```python
from build123d import *

# Parameters (mm, degrees)
SKETCH_1_W                  = 80
SKETCH_1_H                  = 465
EXTRUDE_1_DEPTH             = 107
CUT_EXTRUDE_1_REACH         = 270.152
SKETCH_2_W                  = 45.5
SKETCH_2_H                  = 90
CUT_EXTRUDE_2_REACH         = 270.152
CUT_EXTRUDE_3_REACH         = 261.047
SKETCH_4_R                  = 20
HOLE_WIZARD_M8_1_D          = 6.8
HOLE_WIZARD_M8_1_DEPTH      = 17.25
CUT_EXTRUDE_4_REACH         = 261.047
SKETCH_8_R                  = 9
PATTERN_LINEAR_1_COUNT      = 2
PATTERN_LINEAR_1_PITCH      = 40
PATTERN_LINEAR_1_COUNT_DIR2 = 3
PATTERN_LINEAR_1_PITCH_DIR2 = 110
SKETCH_9_W                  = 80
SKETCH_9_H                  = 20
CUT_EXTRUDE_5_DEPTH         = 6.5
HOLE_WIZARD_M8_2_D          = 6.8
HOLE_WIZARD_M8_2_DEPTH      = 25
HOLE_WIZARD_M8_2_TIP        = 2.042926105
FILLET_1_R                  = 8


with BuildPart() as part:
    # 草图1 → 凸台-拉伸1 (new body)
    with BuildSketch(Plane.XY):
        Rectangle(SKETCH_1_W, SKETCH_1_H)
    extrude(amount=EXTRUDE_1_DEPTH)

    # 草图2 → 切除-拉伸1 (cut, up to next)
    with BuildSketch(Plane.ZY.offset(40), mode=Mode.PRIVATE) as cut_extrude_1_sk1:
        with BuildLine():
            Line((27, 232.5), (27, 115.5))
            ThreePointArc((27, 115.5), (24.656854249, 109.843145751), (19, 107.5))
            Line((19, 107.5), (0, 107.5))
            Line((0, 107.5), (0, 232.5))
            Line((0, 232.5), (27, 232.5))
        make_face()
    cut_extrude_1_tool1 = extrude(cut_extrude_1_sk1.sketch, amount=-CUT_EXTRUDE_1_REACH, mode=Mode.PRIVATE) & part.part
    # 草图2 → 切除-拉伸1 (cut, up to next)
    with BuildSketch(Plane.ZY.offset(40), mode=Mode.PRIVATE) as cut_extrude_1_sk2:
        with Locations((67, 187.5)):
            Rectangle(SKETCH_2_W, SKETCH_2_H)
    cut_extrude_1_tool2 = extrude(cut_extrude_1_sk2.sketch, amount=-CUT_EXTRUDE_1_REACH, mode=Mode.PRIVATE) & part.part
    add(cut_extrude_1_tool1.solids().sort_by_distance((-40, 170.248081, 13.452139))[0], mode=Mode.SUBTRACT)
    add(cut_extrude_1_tool2.solids().sort_by_distance((-40, 187.5, 67))[0], mode=Mode.SUBTRACT)

    # 草图3 → 切除-拉伸2 (cut, up to next)
    with BuildSketch(Plane.ZY.offset(40), mode=Mode.PRIVATE) as cut_extrude_2_sk1:
        Polygon((107, 119.530661885), (61.277191914, 42.311924553), (61.277191914, -232.5), (107, -232.5), align=None)
    cut_extrude_2_tool1 = extrude(cut_extrude_2_sk1.sketch, amount=-CUT_EXTRUDE_2_REACH, mode=Mode.PRIVATE) & part.part
    add(cut_extrude_2_tool1.solids().sort_by_distance((-40, -74.996659, 85.077337))[0], mode=Mode.SUBTRACT)

    # 切除-拉伸3: up to this face of the body (flat: up to its plane)
    cut_extrude_3_end = Plane(part.part.faces().sort_by_distance((0, 174, 27))[0])
    # 草图4 → 切除-拉伸3 (cut, up to the picked face)
    with BuildSketch(Plane.XY.offset(107), mode=Mode.PRIVATE) as cut_extrude_3_sk1:
        with Locations(Location((0, 192.5, 0), (0, 0, 270))):
            Circle(SKETCH_4_R)
    cut_extrude_3_tool1 = split(extrude(cut_extrude_3_sk1.sketch, amount=-CUT_EXTRUDE_3_REACH, mode=Mode.PRIVATE), bisect_by=cut_extrude_3_end, keep=Keep.BOTH, mode=Mode.PRIVATE)
    add(cut_extrude_3_tool1.solids().sort_by(Axis((0, 192.5, 107), (0, 0, -1)))[0], mode=Mode.SUBTRACT)

    # M8 螺纹孔1
    with Locations(Plane.XY.offset(107)):
        with Locations((-25, 162.5), (25, 162.5)):
            Hole(HOLE_WIZARD_M8_1_D / 2, depth=HOLE_WIZARD_M8_1_DEPTH)

    # 草图8 → 切除-拉伸4 (cut, up to next)
    with BuildSketch(Plane(origin=(0, 0, 0), x_dir=(-1, 0, 0), z_dir=(0, 0, -1)), mode=Mode.PRIVATE) as cut_extrude_4_sk1:
        with Locations((-20, 47.5)):
            Circle(SKETCH_8_R)
    cut_extrude_4_tool1 = extrude(cut_extrude_4_sk1.sketch, amount=-CUT_EXTRUDE_4_REACH, mode=Mode.PRIVATE) & part.part
    cut_extrude_4 = cut_extrude_4_tool1.solids().sort_by_distance((20, 47.5, 0))[0]
    add(cut_extrude_4, mode=Mode.SUBTRACT)

    # 阵列(线性)1: Cut-Extrude 4 2 × 3
    with Locations(*[(-i * PATTERN_LINEAR_1_PITCH, -j * PATTERN_LINEAR_1_PITCH_DIR2, 0) for i in range(PATTERN_LINEAR_1_COUNT) for j in range(PATTERN_LINEAR_1_COUNT_DIR2) if (i, j) != (0, 0)]):
        add(cut_extrude_4, mode=Mode.SUBTRACT)

    # 草图9 → 切除-拉伸5 (cut)
    with BuildSketch(Plane(origin=(0, 0, 0), x_dir=(-1, 0, 0), z_dir=(0, 0, -1))):
        with Locations((0, -117.5)):
            Rectangle(SKETCH_9_W, SKETCH_9_H)
    extrude(amount=-CUT_EXTRUDE_5_DEPTH, mode=Mode.SUBTRACT)

    # M8 螺纹孔2
    with Locations(Plane(origin=(0, 0, 6.5), x_dir=(-1, 0, 0), z_dir=(0, 0, -1))):
        with Locations((-20, -117.5), (20, -117.5)):
            Hole(HOLE_WIZARD_M8_2_D / 2, depth=HOLE_WIZARD_M8_2_DEPTH)
            with Locations((0, 0, -(HOLE_WIZARD_M8_2_DEPTH + HOLE_WIZARD_M8_2_TIP / 2))):  # 118° drill point
                Cone(0, HOLE_WIZARD_M8_2_D / 2, HOLE_WIZARD_M8_2_TIP, mode=Mode.SUBTRACT)

    # 圆角1
    fillet_1_edges = [part.edges().sort_by_distance(p)[0] for p in [
        (0, 142.5, 89.75),
        (0, 142.5, 44.25),
    ]]
    fillet(fillet_1_edges, radius=FILLET_1_R)


solid = part.part
```
Design review of the part built by this model. Coordinates are the model's own, in mm. A direction names the side the tool comes from. Give positions to 0.01 mm unless a question says otherwise; leave off trailing zeros. Write each loop counter-clockwise with the first axis right and the second up, starting at its lowest first coordinate (ties: lowest second). Pieces come first, ordered by that corner, then holes. Notation, with made-up numbers: (28, 83.5) - (35, 83.5) arc R30 ccw to (35, 119.5) - close; hole circle Ø1 at (-14, 6). An arc over 180 degrees is marked (long way). Return JSON: item names as keys, results as strings. Group by question number.
(1) Machinability: for faces 1 (the flat face through (-1, 107.5, 10)), 2 (the cylindrical face through (0.56, 144.781, 87.344)), 3 (the cylindrical face through (0.88, 212.48, 35.75)), 4 (the flat face through (-1, -93, 61.277)), 5 (the flat face through (40, -3, 41)), which of the approach directions +Z, -Z, +X, -X, +Y, -Y give a long, thin tool a straight path to every point of the face, cutting with its end or side? Answer none if there is none.
(2) We need section B-B, the plane z = 56.5. Give the boundary of the cut face in (x, y).
(3) To check wall thickness, follow probe 1 along X at (y, z) = (162, 95); probe 2 along Y at (x, z) = (-19.5, 11.5); probe 3 along X at (y, z) = (47.5, 45.5). State the ranges of each line that lie inside material, in increasing order.
(4) We need section A-A, the plane y = 192.5. Give the boundary of the cut face in (x, z), then the cut area to 3 significant figures.
(5) We need section C-C, the plane y = -149. Give the boundary of the cut face in (x, z), then the cut area to 3 significant figures.
(6) Insertion check: pin 1 (23.5 mm diameter, centred on x = -20, y = -62.5, fed in from +Z); pin 2 (8 mm diameter, centred on x = 25, y = 162.5, fed in from -Z); pin 3 (4 mm diameter, centred on x = -25, y = 162.5, fed in from +Z). Each pin has a flat end and moves straight along its axis. Give the tip position at first contact, or say it passes through.
(7) Mouldability with a two-part tool opening along Z and no side actions: class faces 6 (the cylindrical face through (-24.153, -70.485, 30.21)), 7 (the flat face through (-1, 2, 0)), 8 (the cylindrical face through (0.56, 144.906, 46.531)) as +Z half, -Z half, draft (parallel to the pull), parting line (faces both ways), or undercut.
Reported:
{
 "1": {"face 1": "-Z, +X, -X, +Y", "face 2": "+X, -X, +Y", "face 3": "+Z, -Z", "face 4": "+Z, +X, -X, -Y", "face 5": "+Z, -Z, +X, +Y, -Y"},
 "2": {"outline": "(-40, -232.5) - (40, -232.5) - (40, 142.5) - (-40, 142.5) - close; hole circle Ø18 at (-20, -172.5); hole circle Ø18 at (-20, -62.5); hole circle Ø18 at (-20, 47.5); hole circle Ø18 at (20, -172.5); hole circle Ø18 at (20, -62.5); hole circle Ø18 at (20, 47.5)"},
 "3": {"probe 1": "x = -40 to -28.36, -21.64 to 21.64, 28.36 to 40", "probe 2": "y = -232.5 to -181.49, -163.51 to -120.86, -114.14 to -71.49, -53.51 to 38.51, 56.49 to 107.5", "probe 3": "x = -40 to -29, -11 to 11, 29 to 40"},
 "4": {"outline": "(-40, 27) - (-20, 27) - (-20, 44.25) - (-40, 44.25) - close; (-40, 89.75) - (-20, 89.75) - (-20, 107) - (-40, 107) - close; (20, 27) - (40, 27) - (40, 44.25) - (20, 44.25) - close; (20, 89.75) - (40, 89.75) - (40, 107) - (20, 107) - close", "area": "1,380 mm2"},
 "5": {"outline": "(-40, 0) - (40, 0) - (40, 61.28) - (-40, 61.28) - close", "area": "4,900 mm2"},
 "6": {"pin 1": "stops at z = 61.28", "pin 2": "stops at z = 27", "pin 3": "stops at z = 44.25"},
 "7": {"face 6": "draft", "face 7": "-Z half", "face 8": "undercut"}
}
